Check sheet for the modelled part. Datum: model origin and axes. Units: mm. Round coordinates to 2 decimals unless told otherwise and drop trailing zeros. Write each loop counter-clockwise with the first axis right and the second up, starting at its lowest first coordinate (ties: lowest second). Pieces come first, ordered by that corner, then holes. Notation, with made-up numbers: M -9,73 L 13,73 A21 ccw 13,83 Z; hole C 81,20 d5. An arc over 180 degrees is marked long. Put each result on its own line as item: value.
```python
from build123d import *

# Parameters (mm, degrees)
SKETCH1_W           = 101.6
SKETCH1_H           = 101.6
BOSS_EXTRUDE1_DEPTH = 3.175
SKETCH2_R           = 0.99949
CUT_EXTRUDE1_DEPTH  = 3.175
CHAMFER1_SIZE       = 1.27
FILLET1_R           = 2.54


with BuildPart() as part:
    # Sketch1 → Boss-Extrude1 (new body)
    with BuildSketch(Plane(origin=(0, 0, 0), x_dir=(1, 0, 0), z_dir=(0, 1, 0))):
        Rectangle(SKETCH1_W, SKETCH1_H)
    extrude(amount=BOSS_EXTRUDE1_DEPTH)

    # Sketch2 → Cut-Extrude1 (cut)
    with BuildSketch(Plane(origin=(0, 3.175, 0), x_dir=(1, 0, 0), z_dir=(0, 1, 0))):
        with Locations((-38.1, -44.45)):
            Circle(SKETCH2_R)
        with Locations((38.1, -44.45)):
            Circle(SKETCH2_R)
        with Locations((38.1, 44.45)):
            Circle(SKETCH2_R)
        with Locations((-38.1, 44.45)):
            Circle(SKETCH2_R)
    extrude(amount=-CUT_EXTRUDE1_DEPTH, mode=Mode.SUBTRACT)

    # Chamfer1
    chamfer1_edges = [part.edges().sort_by_distance(p)[0] for p in [
        (-39.09949, 0, -44.45),
        (37.10051, 0, -44.45),
        (37.10051, 0, 44.45),
        (-39.09949, 0, 44.45),
    ]]
    chamfer(chamfer1_edges, length=CHAMFER1_SIZE)

    # Fillet1
    fillet1_edges = [part.edges().sort_by_distance(p)[0] for p in [
        (50.8, 3.175, 0),
        (0, 3.175, -50.8),
        (-50.8, 3.175, 0),
        (-50.8, 1.5875, -50.8),
        (50.8, 1.5875, -50.8),
        (50.8, 1.5875, 50.8),
        (-50.8, 1.5875, 50.8),
        (0, 3.175, 50.8),
    ]]
    fillet(fillet1_edges, radius=FILLET1_R)


solid = part.part
```
1. Cross-section at A-A (y = 2.15). Enter the section's corners in (x, z), then the cut area to 3 significant figures.
Computed values:
outline: M -50.3,-48.26 A2.04 ccw -48.26,-50.3 L 48.26,-50.3 A2.04 ccw 50.3,-48.26 L 50.3,48.26 A2.04 ccw 48.26,50.3 L -48.26,50.3 A2.04 ccw -50.3,48.26 Z; hole C -38.1,-44.45 d2; hole C -38.1,44.45 d2; hole C 38.1,-44.45 d2; hole C 38.1,44.45 d2
area: 10,100 mm2
2. Depth check by flat-ended pin: pin 1 Ø1 at (x, y) = (27, 2) entering from +Z; pin 2 Ø1.6 at (x, z) = (38.1, 44.45) entering from +Y. Enter the tip coordinate at first touch or a pass-through.
Computed values:
pin 1: stops at z = 50.65
pin 2: passes through
3. Scan lines: probe 1 along Z at (x, y) = (38.1, 2); probe 2 along Z at (x, y) = (38.1, 2.45); probe 3 along Z at (x, y) = (-39.5, 0.9). Record each from-to range of solid material in increasing order.
Computed values:
probe 1: z = -50.4 to -45.45, -43.45 to 43.45, 45.45 to 50.4
probe 2: z = -50.04 to -45.45, -43.45 to 43.45, 45.45 to 50.04
probe 3: z = -50.79 to 50.79
